Geometry: final body of the model. Coordinates: model frame, mm. Face numbers are marked on the shaded views. A direction names the side the tool comes from. Give positions to 0.01 mm unless a question says otherwise; leave off trailing zeros. Write each loop counter-clockwise with the first axis right and the second up, starting at its lowest first coordinate (ties: lowest second). Pieces come first, ordered by that corner, then holes. Notation, with made-up numbers: M -15.5,-1 L 40.5,-1 A22 ccw 40.5,5 Z; hole C 52.5,4 d1. An arc over 180 degrees is marked long. Use one line per item in the form item = value. Start each with the question number.
Item 1: Section query D-D on y = 5.25. Return loops of the section in (x, z), then the cut area to 3 significant figures.
Item 2: Section query C-C on x = -48. Return loops of the section in (y, z), then the cut area to 3 significant figures.
Item 3: Contact query for flat-ended pins moving along their axis: P1, Ø1.5, axis at x = 6.5, z = 2.5, coming from the +Y side; P2, Ø2.5, axis at y = -9.5, z = 2.5, coming from the -X side. Output: stop coordinate, or through.
Item 4: Material intervals for line 1 along Y through (x, z) = (-56, 2.15); line 2 along Y through (x, z) = (-16, 2.1); line 3 along Y through (x, z) = (-57, 0.2), sorted ascending. Write a range as from..to.
Item 5: Section query B-B on y = -1. Return loops of the section in (x, z), then the cut area to 3 significant figures.
Item 6: Access query for the marked faces 1 and 2. Directions: +Z, -Z, +X, -X, +Y, -Y. A direction counts if a zero-diameter tool reaches every point of the face in a straight line with its end or side. Return the directions, or none.
Item 7: Section query A-A on z = 4.2. Return loops of the section in (x, y), then the cut area to 3 significant figures.
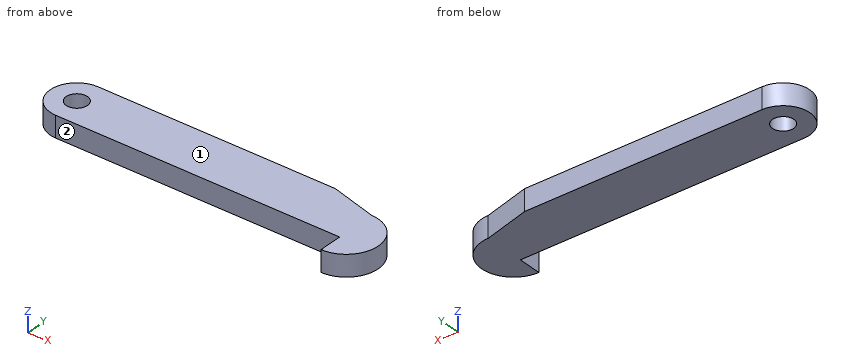
from build123d import *

# Parameters (mm, degrees)
F0_R     = 2.5
F1_DEPTH = 5


with BuildPart() as f1:
    # F0 (on Top) → F1 (new body)
    with BuildSketch(Plane.XY):
        with BuildLine():
            Line((11, 3.25), (0, 6.25))
            Line((0, 6.25), (-56, 6.25))
            ThreePointArc((-56, 6.25), (-62.25, 0), (-56, -6.25))
            Line((-56, -6.25), (11, -6.25))
            Line((11, -6.25), (11, -11.75))
            ThreePointArc((11, -11.75), (18.5, -4.25), (11, 3.25))
        make_face()
        with Locations((-56, 0)):
            Circle(F0_R, mode=Mode.SUBTRACT)
    extrude(amount=F1_DEPTH)


solid = f1.part
Answer sheet:
q1.outline = M -59.39,0 L 3.67,0 L 3.67,5 L -59.39,5 Z
q1.area = 315 mm2
q2.outline = M -6.25,0 L 6.25,0 L 6.25,5 L -6.25,5 Z
q2.area = 62.5 mm2
q3.P1 = 4.68
q3.P2 = 11
q4.line_1 = -6.25..-2.5, 2.5..6.25
q4.line_2 = -6.25..6.25
q4.line_3 = -6.17..-2.29, 2.29..6.17
q5.outline = M -62.17,0 L -58.29,0 L -58.29,5 L -62.17,5 Z; M -53.71,0 L 17.76,0 L 17.76,5 L -53.71,5 Z
q5.area = 377 mm2
q6.face_1 = +Z, +X, -X, +Y, -Y
q6.face_2 = +Z, -Z, -X, -Y
q7.outline = M -56,-6.25 L 11,-6.25 L 11,-11.75 A7.5 ccw 11,3.25 L 0,6.25 L -56,6.25 A6.25 ccw Z; hole C -56,0 d5
q7.area = 951 mm2
